CAD build for the part. Positions are in the model's coordinates, mm. A direction names the side the tool comes from. Give positions to 0.01 mm unless a question says otherwise; leave off trailing zeros. Loops run counter-clockwise (first coordinate to the right, second up) from the corner with the lowest first, then second, coordinate; pieces in that order, holes last.
```python
from build123d import *

# Parameters (mm, degrees)
F1_DEPTH  = 60
F2_T      = -1.6
F4_R      = 3.75
F4_R_2    = 1.25
F4_R_3    = 3.65
F4_R_4    = 3.25
F4_R_5    = 12.75
F4_W      = 71.3
F4_H      = 24.3
F6_DEPTH  = 6.601
F4_R_6    = 13.95
F7_DEPTH  = 1.2
F8_R      = 3.925
F9_DEPTH  = 6.6010001
F8_R_2    = 5.775
F10_DEPTH = 4
F11_DEPTH = 5
F12_W     = 60
F12_H     = 2
F13_DEPTH = 0.8
F14_SIZE  = 0.5


with BuildPart() as f1:
    # F0 (on Right) → F1 (new body, symmetric)
    with BuildSketch(Plane.YZ):
        with BuildLine():
            Line((-21.5, 15), (-21.5, 0))
            Line((-21.5, 0), (21.5, 0))
            Line((21.5, 0), (21.5, 15))
            ThreePointArc((21.5, 15), (18.5710678119, 22.0710678119), (11.5, 25))
            Line((11.5, 25), (-11.5, 25))
            ThreePointArc((-11.5, 25), (-18.5710678119, 22.0710678119), (-21.5, 15))
        make_face()
    extrude(amount=F1_DEPTH, both=True)

    # F2
    f2_openings = [f1.faces().sort_by_distance(p)[0] for p in [
        (0, 0, 0),
    ]]
    offset(amount=F2_T, openings=f2_openings)

    # F4 (on offset) → F5 (join, up to the next surface of F1)
    with BuildSketch(Plane(origin=(0, 0, 18.4), x_dir=(1, 0, 0), z_dir=(0, 0, -1))):
        with Locations((53.4, -15.5)):
            Circle(F4_R)
        with Locations((53.4, -15.5)):
            Circle(F4_R_2, mode=Mode.SUBTRACT)
        with Locations((53.4, 15.5)):
            Circle(F4_R_3)
        with Locations((53.4, 15.5)):
            Circle(F4_R_2, mode=Mode.SUBTRACT)
        with Locations((-21.6, -15.5)):
            Circle(F4_R)
        with Locations((-21.6, -15.5)):
            Circle(F4_R_2, mode=Mode.SUBTRACT)
        with Locations((-21.6, 15.5)):
            Circle(F4_R_4)
        with Locations((-21.6, 15.5)):
            Circle(F4_R_2, mode=Mode.SUBTRACT)
    extrude(until=Until.NEXT, dir=(0, 0, 1))

    # F4 (on offset) → F6 (cut, through all)
    with BuildSketch(Plane(origin=(0, 0, 18.4), x_dir=(1, 0, 0), z_dir=(0, 0, -1))):
        with Locations((-41.8, 0)):
            Circle(F4_R_5)
        with Locations((15.9, 0)):
            Rectangle(F4_W, F4_H)
    extrude(amount=-F6_DEPTH, mode=Mode.SUBTRACT)



with BuildPart() as f7:
    # F4 (on offset) → F7 (new body)
    with BuildSketch(Plane(origin=(0, 0, 18.4), x_dir=(1, 0, 0), z_dir=(0, 0, -1))):
        with Locations((-41.8, 0)):
            Circle(F4_R_6)
        with Locations((-41.8, 0)):
            Circle(F4_R_5, mode=Mode.SUBTRACT)
        with Locations((-41.8, 0)):
            Circle(F4_R_5)
    extrude(amount=-F7_DEPTH)

    # F8 (on face) → F9 (cut, through all)
    with BuildSketch(Plane(origin=(0, 0, 18.4), x_dir=(1, 0, 0), z_dir=(0, 0, -1))):
        with Locations((-41.8, 0)):
            Circle(F8_R)
    extrude(amount=-F9_DEPTH, mode=Mode.SUBTRACT)

    # F8 (on face) → F10 (join)
    with BuildSketch(Plane(origin=(0, 0, 18.4), x_dir=(1, 0, 0), z_dir=(0, 0, -1))):
        with Locations((-41.8, 0)):
            Circle(F8_R_2)
        with Locations((-41.8, 0)):
            Circle(F8_R, mode=Mode.SUBTRACT)
    extrude(amount=-F10_DEPTH)


with BuildPart() as f1_1:
    add(f1.part)

    add(f7.part)  # F11 merges F7
    # F4 (on offset) → F11 (join, through all)
    with BuildSketch(Plane(origin=(0, 0, 18.4), x_dir=(1, 0, 0), z_dir=(0, 0, -1))):
        with Locations((-41.8, 0)):
            Circle(F4_R_6)
        with Locations((-41.8, 0)):
            Circle(F4_R_5, mode=Mode.SUBTRACT)
    extrude(amount=-F11_DEPTH)


with BuildPart() as f13:
    # F12 (on face) → F13 (new body)
    with BuildSketch(Plane.XZ.offset(-19.9)):
        with Locations((0, 6)):
            Rectangle(F12_W, F12_H)
    extrude(amount=-F13_DEPTH)

    # F14
    f14_edges = [f13.edges().sort_by_distance(p)[0] for p in [
        (0, 20.7, 5),
        (0, 20.7, 7),
    ]]
    chamfer(f14_edges, length=F14_SIZE)


with BuildPart() as f15_1:
    # F15: instance of F13
    add(f13.part.mirror(Plane.XZ))


with BuildPart() as f1_2:
    add(f1_1.part)

    # F16: cut F13, F15_1
    add(f13.part, mode=Mode.SUBTRACT)
    add(f15_1.part, mode=Mode.SUBTRACT)


solid = f1_2.part
```
1. Probe line 1 along Y through (x, z) = (53.4, 20.45); line 2 along X through (y, z) = (-15.5, 19.95); line 3 along X through (y, z) = (-13, 11.5). List the from-to ranges inside material, lowest first.
Responses:
line 1: y = -19.88 to -16.75, -14.25 to -11.85, 11.75 to 14.25, 16.75 to 19.88
line 2: x = -60 to -58.4, -24.85 to -22.85, -20.35 to -18.35, 49.75 to 52.15, 54.65 to 57.05, 58.4 to 60
line 3: x = -60 to -58.4, 58.4 to 60
2. Pull direction X, two halves, no side cores. Call faces 1 (the face through (-60, 0, 13)), 2 (the face through (1, -21.5, 8)), 3 (the face through (0.818, -17.374, 21.005)): released by +X, released by -X, zero draft, split by the parting line, or undercut.
Responses:
face 1: released by -X
face 2: zero draft
face 3: undercut
3. Tool access for faces 4 (the face through (-58.4, 0, 12)), 5 (the face through (0.84, -18.49, 22.15)): list every direction of +Z, -Z, +X, -X, +Y, -Y with a clear straight run to the whole face (end or side of a thin tool).
Responses:
face 4: -Z
face 5: +Z, +X, -X, -Y
4. Saw through at D-D, the plane y = -15.5. List the corners of the cut face in (x, z), and give its area (3 significant figures).
Responses:
outline: (-60, 0) - (-58.4, 0) - (-58.4, 22.39) - (-24.85, 22.39) - (-24.85, 18.4) - (-22.85, 18.4) - (-22.85, 22.39) - (-20.35, 22.39) - (-20.35, 18.4) - (-18.35, 18.4) - (-18.35, 22.39) - (49.75, 22.39) - (49.75, 18.4) - (52.15, 18.4) - (52.15, 22.39) - (54.65, 22.39) - (54.65, 18.4) - (57.05, 18.4) - (57.05, 22.39) - (58.4, 22.39) - (58.4, 0) - (60, 0) - (60, 24.17) - (-60, 24.17) - close
area: 320 mm2
5. Saw through at B-B, the plane y = 0. List the corners of the cut face in (x, z) (3 decimals), and give its area (3 significant figures).
Responses:
outline: (-60, 0) - (-58.4, 0) - (-58.4, 23.4) - (-55.75, 23.4) - (-55.75, 18.4) - (-45.725, 18.4) - (-45.725, 22.4) - (-47.575, 22.4) - (-47.575, 19.6) - (-54.55, 19.6) - (-54.55, 25) - (-60, 25) - close; (-37.875, 18.4) - (-27.85, 18.4) - (-27.85, 23.4) - (-19.75, 23.4) - (-19.75, 25) - (-29.05, 25) - (-29.05, 19.6) - (-36.025, 19.6) - (-36.025, 22.4) - (-37.875, 22.4) - close; (51.55, 23.4) - (58.4, 23.4) - (58.4, 0) - (60, 0) - (60, 25) - (51.55, 25) - close
area: 156 mm2
6. Saw through at A-A, the plane z = 9.25. List the corners of the cut face in (x, y).
Responses:
outline: (-60, -21.5) - (60, -21.5) - (60, 21.5) - (-60, 21.5) - close; hole (-58.4, -19.9) - (58.4, -19.9) - (58.4, 19.9) - (-58.4, 19.9) - close
7. Saw through at C-C, the plane x = -41.8. List the corners of the cut face in (y, z) (3 decimals).
Responses:
outline: (-21.5, 0) - (-19.9, 0) - (-19.9, 15) arc R8.4 cw to (-13.95, 23.035) - (-13.95, 18.4) - (-3.925, 18.4) - (-3.925, 22.4) - (-5.775, 22.4) - (-5.775, 19.6) - (-12.75, 19.6) - (-12.75, 24.922) arc R10 ccw to (-21.5, 15) - close; (3.925, 18.4) - (13.95, 18.4) - (13.95, 23.035) arc R8.4 cw to (19.9, 15) - (19.9, 0) - (21.5, 0) - (21.5, 15) arc R10 ccw to (12.75, 24.922) - (12.75, 19.6) - (5.775, 19.6) - (5.775, 22.4) - (3.925, 22.4) - close
8. Drop flat-ended pins along their axis: pin 1 (3 mm diameter, centred on x = 1, y = 10, fed in from -Z); pin 2 (2 mm diameter, centred on x = 53.4, y = 15.5, fed in from +Z); pin 3 (2 mm diameter, centred on x = 53.4, y = -15.5, fed in from -Z); pin 4 (6 mm diameter, centred on x = -39.5, y = 2.5, fed in from +Z). Give the stop position or say it passes through.
Responses:
pin 1: passes through
pin 2: stops at z = 24.54
pin 3: stops at z = 21.75
pin 4: stops at z = 22.4
